Drawing for the job (mm, zero at the part's lowest x, y, z). Give positions to 0.01 mm unless a question says otherwise; leave off trailing zeros. Order: outer loops, then holes, each group sorted by start corner. A loop starts at its lowest first (then second) coordinate and runs counter-clockwise, first axis right, second up. Notation, with made-up numbers: (66.5, -2.75) -> (124.5, -2.75) arc R37 cw to (124.5, 33.25) -> close; hole circle Ø8 at (-38, -9). An arc over 180 degrees is marked (long way). One line per item, written item: value. Start each with the question number.
(1) Saw through at C-C on z = 38.5. Give the cut face in (x, y), plus the area to 3 significant figures.
(2) Pin check, flat tip, straight feed: pin 1 (1 mm diameter, centred on x = 92.5, y = 0.5, fed in from -Z). Stop position of the tip, or through.
(3) Saw through at A-A on y = 0.5. Give the cut face in (x, z), plus the area to 3 significant figures.
(4) Probe line 1 (X direction, y = 1.5, z = 103) (1 decimal); line 2 (Z direction, x = 31, y = 1.6); line 3 (X direction, y = 1.3, z = 24) (1 decimal). List the from-to ranges inside material, lowest first.
(5) Saw through at B-B on x = 46. Give the cut face in (y, z), plus the area to 3 significant figures.
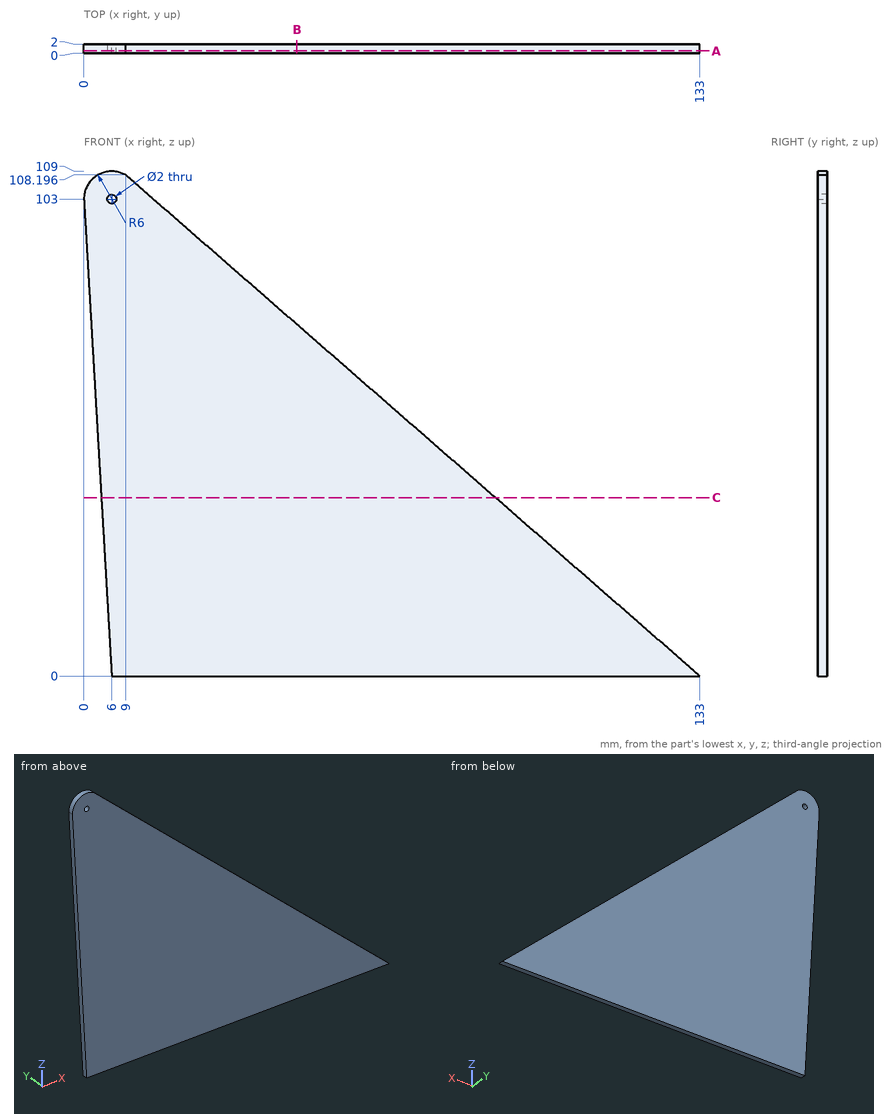
Results below:
1. outline: (3.76, 0) -> (88.88, 0) -> (88.88, 2) -> (3.76, 2) -> close
1. area: 170 mm²
2. pin 1: stops at z = 0
3. outline: (0, 103) -> (6, 0) -> (133, 0) -> (9, 108.2) arc R6 ccw to start; hole circle Ø2 at (6, 103)
3. area: 7,370 mm²
4. line 1: x = 0 to 5, 7 to 15
4. line 2: z = 0 to 89
4. line 3: x = 4.6 to 105.5
5. outline: (0, 0) -> (2, 0) -> (2, 75.91) -> (0, 75.91) -> close
5. area: 152 mm²
